```python
from build123d import *


# Read off the part's stored shape, not the designer's step: Shell2
with BuildPart() as part:
    # Sketch1 → Revolve1 (revolve)
    with BuildSketch(Plane.XY, mode=Mode.PRIVATE) as revolve1_sk:
        with BuildLine():
            Line((-8.7376, 0), (-8.7376, 0.127))
            Line((-8.7376, 0.127), (-7.830223739, 3.559760253))
            ThreePointArc((-7.830223739, 3.559760253), (-7.323100489, 4.047695704), (-6.656513532, 3.822048141))
            Line((-6.656513532, 3.822048141), (-3.556, 0.127))
            Line((-3.556, 0.127), (-3.556, 0))
            Line((-3.556, 0), (-8.7376, 0))
        make_face()
    revolve(revolve1_sk.sketch.rotate(Axis((0, 0, 0), (0, 1, 0)), 270), axis=Axis((0, 0, 0), (0, 1, 0)))

    # Shell2 outline → Shell2 (revolve, cut)
    with BuildSketch(Plane.XY):
        Polygon((7.120216638, 3.139812195), (4.485601383, 0), (7.94385, 0), (7.94385, 0.023865712), align=None)
    revolve(axis=Axis((0, 0, 0), (0, 1, 0)), mode=Mode.SUBTRACT)


solid = part.part
```
Read the model definition and answer for the solid it produces. Units are mm, in the model's axes. Give positions to 0.01 mm unless a question says otherwise; leave off trailing zeros. Write each loop counter-clockwise with the first axis right and the second up, starting at its lowest first coordinate (ties: lowest second). Pieces come first, ordered by that corner, then holes. Notation, with made-up numbers: M 13.25,-6 L 26.25,-6 A30 ccw 26.25,28 Z; hole C 3,80 d8. An arc over 180 degrees is marked long. Put each result on its own line as item: value. Start each with the question number.
1. The part is cut by section C-C, the plane y = 1.95. Give the vertices of the cut face in (x, z).
2. The part is cut by section D-D, the plane y = 2.9. Give the vertices of the cut face in (x, z).
3. Consider line 1 along X through (y, z) = (0.05, 0); line 2 along X through (y, z) = (0.5, -1.5); line 3 along Z through (x, y) = (-2.5, 0.65). Determine where each line is inside the solid, lowest interval first.
4. For a pull along X with two mould halves and no side action, classify faces 1 (the conical face through (-3.661, 0.152, 2.807)), 2 (the flat face through (8, 0, 2)), 3 (the conical face through (7.687, 3.393, 1.707)) as released by +X, released by -X, zero draft, split by the parting line, or undercut.
5. Each of these flat-tipped pins is pushed along its axis until it touches: pin 1 Ø4 at (x, z) = (4.5, -5.5) entering from -Y; pin 2 Ø2 at (x, y) = (-1.5, 3) entering from +Z; pin 3 Ø5.5 at (x, z) = (0, 0) entering from -Y. Where does it stop, or does it pass through?
Final values:
1. outline: C 0,0 d16.51; C 0,0 d12.24; hole C 0,0 d14.87; hole C 0,0 d10.17
2. outline: C 0,0 d16.01; C 0,0 d13.84; hole C 0,0 d14.37; hole C 0,0 d11.77
3. line 1: x = -8.74 to -7.94, -4.53 to -3.56, 3.56 to 4.53, 7.94 to 8.74
3. line 2: x = -8.51 to -7.67, -4.67 to -3.57, 3.57 to 4.67, 7.67 to 8.51
3. line 3: z = -8.23 to -7.37, -4.37 to -3.12, 3.12 to 4.37, 7.37 to 8.23
4. face 1: undercut
4. face 2: zero draft
4. face 3: split by the parting line
5. pin 1: stops at y = 0
5. pin 2: stops at z = 8.15
5. pin 3: passes through
